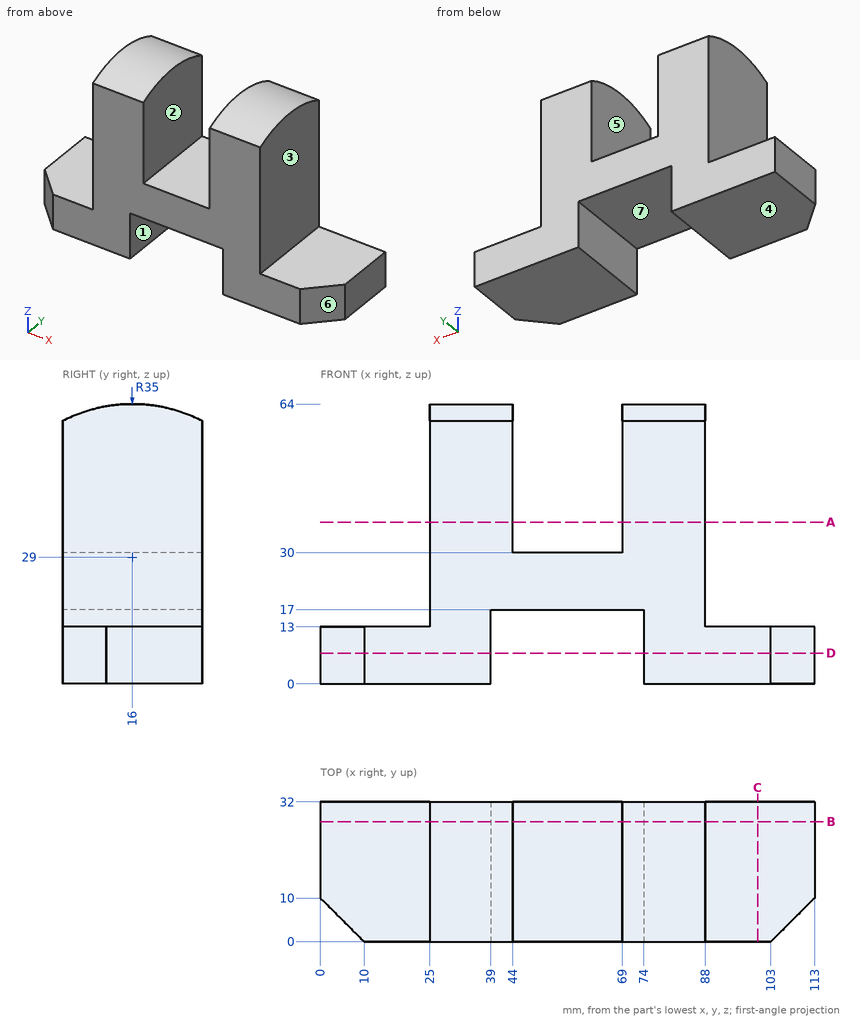
The figure shows three views and two pictorial views of one solid part (mm, origin at its lowest corner). Answer the questions. A direction names the side the tool comes from. Round coordinates to 2 decimals unless told otherwise and drop trailing zeros. Loops run counter-clockwise (first coordinate to the right, second up) from the corner with the lowest first, then second, coordinate; pieces in that order, holes last. Notation, with made-up numbers: (49.5, 57) -> (97.5, 57) arc R26 cw to (97.5, 78) -> close; hole circle Ø5 at (32, 32). An arc over 180 degrees is marked (long way). Use one line per item in the form item = value.
(1) Find section C-C on x = 100. Give the vertices of the cut face in (y, z), then the cut area to 3 significant figures.
Answer list:
outline = (0, 0) -> (32, 0) -> (32, 13) -> (0, 13) -> close
area = 416 mm2
(2) Straight lines are drawn through the part: line 1 (X direction, y = 27, z = 49); line 2 (Z direction, x = 8.5, y = 13.5); line 3 (X direction, y = 7.5, z = 6). For each, find the intervals that lie inside material, in ascending order.
Answer list:
line_1 = 25 to 44, 69 to 88
line_2 = 0 to 13
line_3 = 2.5 to 39, 74 to 110.5
(3) A tool of negligible diameter and unlimited length cuts with its end or side. For the marked faces 1, 2 and 3, from which of +Z, -Z, +X, -X, +Y, -Y can it reach the whole face along a straight path? Write none if from no direction.
Answer list:
face_1 = -Z, +Y, -Y
face_2 = +Z, +Y, -Y
face_3 = +Z, +X, +Y, -Y
(4) For a pull along X with two mould halves and no side action, classify the marked faces 4, 5, 6 and 7 as released by +X, released by -X, zero draft, split by the parting line, or undercut.
Answer list:
face_4 = zero draft
face_5 = undercut
face_6 = released by +X
face_7 = undercut
(5) Find section B-B on y = 27.5. Give the vertices of the cut face in (x, z).
Answer list:
outline = (0, 0) -> (39, 0) -> (39, 17) -> (74, 17) -> (74, 0) -> (113, 0) -> (113, 13) -> (88, 13) -> (88, 62.06) -> (69, 62.06) -> (69, 30) -> (44, 30) -> (44, 62.06) -> (25, 62.06) -> (25, 13) -> (0, 13) -> close
(6) Find section D-D on z = 7. Give the vertices of the cut face in (x, y).
Answer list:
outline = (0, 10) -> (10, 0) -> (39, 0) -> (39, 32) -> (0, 32) -> close; (74, 0) -> (103, 0) -> (113, 10) -> (113, 32) -> (74, 32) -> close
(7) Flat-ended cylindrical pins translate along their axes: P1, Ø9.5, axis at x = 61, y = 10, coming from the -Z side; P2, Ø1, axis at y = 16, z = 20, coming from the +X side; P3, Ø3, axis at x = 61.5, y = 13.5, coming from the +Z side. Find the tip coordinate at first contact, or state that the pin passes through.
Answer list:
P1 = 17
P2 = 88
P3 = 30
(8) Find section A-A on z = 37. Give the vertices of the cut face in (x, y).
Answer list:
outline = (25, 0) -> (44, 0) -> (44, 32) -> (25, 32) -> close; (69, 0) -> (88, 0) -> (88, 32) -> (69, 32) -> close
